Here's how the part is built. I have some questions about the finished solid (model axes, mm). A direction names the side the tool comes from. Round coordinates to 2 decimals unless told otherwise and drop trailing zeros. Loops run counter-clockwise (first coordinate to the right, second up) from the corner with the lowest first, then second, coordinate; pieces in that order, holes last. Notation, with made-up numbers: M 31,-14 L 39,-14 A21 ccw 39,1 Z; hole C 12,88.25 d5. An arc over 180 degrees is marked long. Use a Markdown table: item, result.
```python
from build123d import *

# Parameters (mm, degrees)
F0_R     = 3.175
F1_DEPTH = 44.45
F2_W     = 34.925
F2_H     = 40.217792
F3_DEPTH = 76.201


with BuildPart() as f1:
    # F0 (on Front) → F1 (new body)
    with BuildSketch(Plane.XZ):
        with BuildLine():
            Line((0, 23.8125), (0, 0))
            Line((0, 0), (76.2, 0))
            Line((76.2, 0), (76.2, 23.8125))
            ThreePointArc((76.2, 23.8125), (70.620384, 37.282884), (57.15, 42.8625))
            Line((57.15, 42.8625), (19.05, 42.8625))
            ThreePointArc((19.05, 42.8625), (5.579616, 37.282884), (0, 23.8125))
        make_face()
        with Locations((38.1, 31.75)):
            Circle(F0_R, mode=Mode.SUBTRACT)
    extrude(amount=F1_DEPTH)

    # F2 (on face) → F3 (cut, through all)
    with BuildSketch(Plane.YZ.offset(76.2)):
        with Locations((-22.225, 24.871396)):
            Rectangle(F2_W, F2_H)
    extrude(amount=-F3_DEPTH, mode=Mode.SUBTRACT)


solid = f1.part
```
Q1. For faces 4 (the flat face through (38, -22, 0)), 5 (the flat face through (39, -4.763, 24)), which set-ups out of +Z, -Z, +X, -X, +Y, -Y let a thin tool reach every point of the face, with its end or its side?
Return value:
| item | result |
|---|---|
| face 4 | -Z, +X, -X, +Y, -Y |
| face 5 | +Z, +X, -X |
Q2. Imagine slicing it at B-B, the plane z = 17. Please give me the cut outline in (x, y), then the cut area to 3 significant figures.
Return value:
| item | result |
|---|---|
| outline | M 0,-44.45 L 76.2,-44.45 L 76.2,-39.69 L 0,-39.69 Z; M 0,-4.76 L 76.2,-4.76 L 76.2,0 L 0,0 Z |
| area | 726 mm^2 |
Q3. Imagine slicing it at A-A, the plane x = 38.1. Give the number of separate pieces and of enclosed holes in the cut face, then the cut area to 3 significant figures.
Return value:
| item | result |
|---|---|
| separate pieces | 3 |
| enclosed holes | 0 |
| area | 514 mm^2 |
Q4. Imagine slicing it at D-D, the plane x = 27. Please give me the cut outline in (y, z).
Return value:
| item | result |
|---|---|
| outline | M -44.45,0 L 0,0 L 0,42.86 L -4.76,42.86 L -4.76,4.76 L -39.69,4.76 L -39.69,42.86 L -44.45,42.86 Z |
Q5. I need wall thicknesses on line 1 (Y direction, x = 8.5, z = 32.5); line 2 (Z direction, x = 38.1, y = -42.45) (1 decimal); line 3 (Z direction, x = 26.5, y = -25). Which ranges of each line are inside material? Lowest first, please. Write a range as from..to.
Return value:
| item | result |
|---|---|
| line 1 | y = -44.45..-39.69, -4.76..0 |
| line 2 | z = 0..28.6, 34.9..42.9 |
| line 3 | z = 0..4.76 |
Q6. Will these pins go through, and if not, where does the flat tip stop? P1, Ø4, axis at x = 8.5, y = -8.5, coming from the +Z side; P2, Ø5, axis at x = 38.1, z = 31.75, coming from the +Y side.
Return value:
| item | result |
|---|---|
| P1 | stops at z = 4.76 |
| P2 | passes through |
Q7. We'd pull the mould along Z, two halves only. Please class faces 1 (the flat face through (76.2, -22, 4)), 2 (the cylindrical face through (37.41, -42.04, 28.65)), 3 (the flat face through (39, -22, 4.762)): pulls with the +Z half, pulls with the -Z half, needs draft (parallel to the pull), parting line crosses it, or undercut.
Return value:
| item | result |
|---|---|
| face 1 | needs draft |
| face 2 | undercut |
| face 3 | pulls with the +Z half |
